Geometry check sheet. Reference: the model listing, model coordinates, mm. Give positions to 0.01 mm unless a question says otherwise; leave off trailing zeros. Loops run counter-clockwise (first coordinate to the right, second up) from the corner with the lowest first, then second, coordinate; pieces in that order, holes last. Notation, with made-up numbers: (-30, 59) -> (7, 59) arc R12 ccw to (7, 66) -> close; hole circle Ø2 at (85, -39). An arc over 180 degrees is marked (long way). Write item = value, one per line. Start each with the question number.
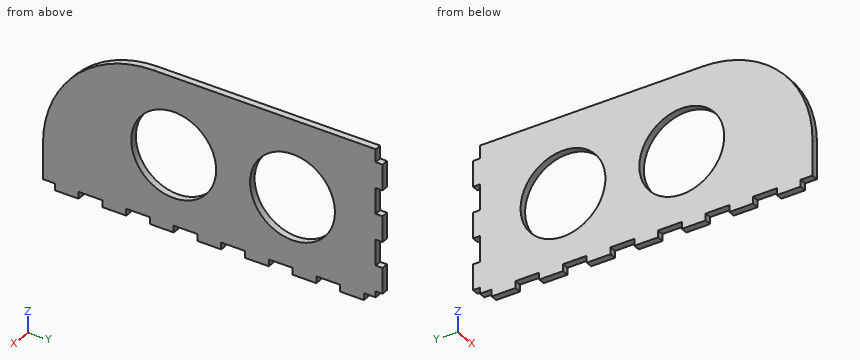
```python
from build123d import *

# Parameters (mm, degrees)
SKETCH071_W     = 200
SKETCH071_H     = 90
PAD035_DEPTH    = 4
SKETCH070_R     = 25
SKETCH070_W     = 7
SKETCH070_H     = 4
SKETCH070_W_2   = 14
SKETCH070_W_3   = 4
SKETCH070_H_2   = 15
SKETCH070_H_3   = 7.5
POCKET031_DEPTH = 4
FILLET002_R     = 65


with BuildPart() as part:
    # Sketch071 → Pad035 (new body)
    with BuildSketch(Plane.YZ):
        Rectangle(SKETCH071_W, SKETCH071_H)
    extrude(amount=PAD035_DEPTH)

    # Sketch070 (on Face6 of Pad035) → Pocket031 (cut)
    with BuildSketch(Plane.YZ.offset(4)):
        with Locations((-23, 0)):
            Circle(SKETCH070_R)
        with Locations((47, 0)):
            Circle(SKETCH070_R)
        with Locations((-96.5, -43)):
            Rectangle(SKETCH070_W, SKETCH070_H)
        with Locations((-72, -43)):
            Rectangle(SKETCH070_W_2, SKETCH070_H)
        with Locations((-44, -43)):
            Rectangle(SKETCH070_W_2, SKETCH070_H)
        with Locations((-16, -43)):
            Rectangle(SKETCH070_W_2, SKETCH070_H)
        with Locations((12, -43)):
            Rectangle(SKETCH070_W_2, SKETCH070_H)
        with Locations((40, -43)):
            Rectangle(SKETCH070_W_2, SKETCH070_H)
        with Locations((68, -43)):
            Rectangle(SKETCH070_W_2, SKETCH070_H)
        with Locations((98, -15)):
            Rectangle(SKETCH070_W_3, SKETCH070_H_2)
        with Locations((98, 15)):
            Rectangle(SKETCH070_W_3, SKETCH070_H_2)
        with Locations((98, 41.25)):
            Rectangle(SKETCH070_W_3, SKETCH070_H_3)
        Polygon((89, -45), (89, -41), (96, -41), (96, -37.5), (100, -37.5), (100, -45), align=None)
    extrude(amount=-POCKET031_DEPTH, mode=Mode.SUBTRACT)

    # Fillet002
    fillet002_edges = [part.edges().sort_by_distance(p)[0] for p in [
        (2, -100, 45),
    ]]
    fillet(fillet002_edges, radius=FILLET002_R)


with BuildPart() as part_1:
    # Body035 placement: moved
    add(part.part.moved(Location((-331, -402, 0))))


solid = part_1.part
```
1) Section check C-C (x = -328). Give the number of separate pieces and of enclosed holes in the cut face, plus the area to 3 significant figures.
2) Section check B-B (y = -335.5). Enter the section's corners in (x, z).
3) Section check A-A (z = 0). Enter the section's corners in (x, y), plus the area to 3 significant figures.
4) Thickness scan on line 1 (Y direction, x = -329.1, z = -14.5); line 2 (Z direction, x = -328.3, y = -416); line 3 (Z direction, x = -328.25, y = -427). Record the ranges inside material, lowest first.
5) Depth check by flat-ended pin: pin 1 Ø2 at (x, z) = (-329, 13.5) entering from +Y; pin 2 Ø1.2 at (x, z) = (-330, -43.5) entering from +Y; pin 3 Ø1.2 at (x, z) = (-329.5, -42.5) entering from -Y. Enter the tip coordinate at first touch or a pass-through.
Check result:
q1.separate_pieces = 1
q1.enclosed_holes = 2
q1.area = 12,600 mm2
q2.outline = (-331, -41) -> (-327, -41) -> (-327, -15.64) -> (-331, -15.64) -> close; (-331, 15.64) -> (-327, 15.64) -> (-327, 45) -> (-331, 45) -> close
q3.outline = (-331, -498.85) -> (-327, -498.85) -> (-327, -450) -> (-331, -450) -> close; (-331, -400) -> (-327, -400) -> (-327, -380) -> (-331, -380) -> close; (-331, -330) -> (-327, -330) -> (-327, -302) -> (-331, -302) -> close
q3.area = 387 mm2
q4.line_1 = -501.77 to -445.37, -404.63 to -375.37, -334.63 to -306
q4.line_2 = -41 to -23.32, 23.32 to 45
q4.line_3 = -45 to -24.92, 24.92 to 45
q5.pin_1 = -306
q5.pin_2 = -313
q5.pin_3 = -495
